The listing builds one solid part. Answer for the finished solid, in the listing's coordinates (mm). A direction names the side the tool comes from. Round coordinates to 2 decimals unless told otherwise and drop trailing zeros. Write each loop counter-clockwise with the first axis right and the second up, starting at its lowest first coordinate (ties: lowest second). Pieces come first, ordered by that corner, then holes. Notation, with made-up numbers: M 87,60 L 92,60 A27 cw 92,85 Z; hole C 11.25,-22.75 d6. An arc over 180 degrees is marked long. One line per item, written item: value. Start each with the question number.
(1) Given P1, Ø1.5, axis at y = 3.5, z = -3, coming from the +X side; P2, Ø1.5, axis at x = 1.5, z = -1, coming from the +Y side, each flat-ended and moving along its own axis, determine where each tip first touches the part or whether it passes through.
(2) Section A-A (z = -3.8) is taken. Determine the outline of the cut face in (x, y), plus the area to 3 significant figures.
(3) Section B-B (x = -0.3) is taken. Determine the outline of the cut face in (y, z).
(4) For faces 1 (the flat face through (-1.5, 1.5, -2)), 2 (the flat face through (2, 3, -3)), 3 (the flat face through (-2, 3, -3)), determine the directions among +Z, -Z, +X, -X, +Y, -Y from which every point of the face is accessible in a straight line to the end or side of a thin tool.
(5) Section D-D (z = -1.4) is taken. Determine the outline of the cut face in (x, y), plus the area to 3 significant figures.
(6) Consider probe 1 along Y at (x, z) = (-2.2, -3.35); probe 2 along X at (y, z) = (4.1, -1.45) (3 decimals); probe 3 along Z at (x, y) = (1.25, 3.35). Determine where each line is inside the solid, lowest interval first.
(7) Section C-C (y = 3.5) is taken. Determine the outline of the cut face in (x, z).
```python
from build123d import *

# Parameters (mm, degrees)
BOSS_EXTRUDE1_DEPTH = 3
BOSS_EXTRUDE2_DEPTH = 2


with BuildPart() as part:
    # Sketch1 → Boss-Extrude1 (new body)
    with BuildSketch(Plane(origin=(0, 0, 0), x_dir=(1, 0, 0), z_dir=(0, 1, 0))):
        Polygon((0, 0), (-3, 4), (3, 4), align=None)
    extrude(amount=BOSS_EXTRUDE1_DEPTH)

    # Sketch2 → Boss-Extrude2 (add)
    with BuildSketch(Plane(origin=(0, 3, 0), x_dir=(1, 0, 0), z_dir=(0, 1, 0))):
        Polygon((0, 0), (-2, 4), (2, 4), align=None)
    extrude(amount=BOSS_EXTRUDE2_DEPTH)


solid = part.part
```
Recorded:
1. P1: stops at x = 2.67
1. P2: stops at y = 3
2. outline: M -2.85,0 L 2.85,0 L 2.85,3 L 1.9,3 L 1.9,5 L -1.9,5 L -1.9,3 L -2.85,3 Z
2. area: 24.7 mm2
3. outline: M 0,-4 L 5,-4 L 5,-0.6 L 3,-0.6 L 3,-0.4 L 0,-0.4 Z
4. face 1: +Z, -X, +Y, -Y
4. face 2: +Z, +X, +Y
4. face 3: +Z, -X, +Y
5. outline: M -1.05,0 L 1.05,0 L 1.05,3 L 0.7,3 L 0.7,5 L -0.7,5 L -0.7,3 L -1.05,3 Z
5. area: 9.10 mm2
6. probe 1: y = 0 to 3
6. probe 2: x = -0.725 to 0.725
6. probe 3: z = -4 to -2.5
7. outline: M -2,-4 L 2,-4 L 0,0 Z
